Work out the finished part from the listing and answer in its coordinate system (mm). A direction names the side the tool comes from. Round coordinates to 2 decimals unless told otherwise and drop trailing zeros. Write each loop counter-clockwise with the first axis right and the second up, starting at its lowest first coordinate (ties: lowest second). Pieces come first, ordered by that corner, then holes.
from build123d import *

# Parameters (mm, degrees)
ESQUISSE1_R             = 1.6
BOSS_EXTRU_1_DEPTH      = 10.1
ESQUISSE2_R             = 32.8
BOSS_EXTRU_2_DEPTH      = 21
ENL_V_MAT_EXTRU_1_DEPTH = 3.5
ESQUISSE4_R             = 32.8
BOSS_EXTRU_3_DEPTH      = 3.5
ESQUISSE5_R             = 16
BOSS_EXTRU_4_DEPTH      = 20.7
ESQUISSE8_R             = 5
BOSS_EXTRU_7_DEPTH      = 5.5
SKETCH6_R               = 34.35
BOSS_EXTRUDE3_DEPTH     = 9.3
CUT_EXTRUDE1_REACH      = 83.139
CUT_EXTRUDE1_END_RADIUS = 32.8
SKETCH5_R               = 5.25
ESQUISSE6_R             = 1
BOSS_EXTRU_5_DEPTH      = 7.7
BOSS_EXTRUDE4_DEPTH     = 10.6


with BuildPart() as part:
    # Esquisse1 → Boss.-Extru.1 (new body)
    with BuildSketch(Plane.XY):
        with BuildLine():
            ThreePointArc((-56.3, -16.861494596), (-60.528670487, -14.599558136), (-64.01, -11.301322931))
            ThreePointArc((-64.01, -11.301322931), (-65, 0), (-64.01, 11.301322931))
            ThreePointArc((-64.01, 11.301322931), (-60.528670487, 14.599558136), (-56.3, 16.861494596))
            Line((-56.3, 16.861494596), (-39.156313776, 23.266930519))
            ThreePointArc((-39.156313776, 23.266930519), (-36.515940127, 29.057304168), (-30.725566478, 26.416930519))
            Line((-30.725566478, 26.416930519), (-12.425, 33.254614341))
            ThreePointArc((-12.425, 33.254614341), (1.381675102, 35.473102119), (14.973963383, 32.187426436))
            Line((14.973963383, 32.187426436), (20.756023105, 34.801647207))
            ThreePointArc((20.756023105, 34.801647207), (24.347774736, 34.238511045), (26, 31))
            Line((26, 31), (25.359978077, 24.841930519))
            ThreePointArc((25.359978077, 24.841930519), (35.5, 0), (25.359978077, -24.841930519))
            Line((25.359978077, -24.841930519), (26, -31))
            ThreePointArc((26, -31), (24.347774736, -34.238511045), (20.756023105, -34.801647207))
            Line((20.756023105, -34.801647207), (14.973963383, -32.187426436))
            ThreePointArc((14.973963383, -32.187426436), (1.381675102, -35.473102119), (-12.425, -33.254614341))
            Line((-12.425, -33.254614341), (-30.725566478, -26.416930519))
            ThreePointArc((-30.725566478, -26.416930519), (-36.515940127, -29.057304168), (-39.156313776, -23.266930519))
            Line((-39.156313776, -23.266930519), (-56.3, -16.861494596))
        make_face()
        with Locations((-35, -25)):
            Circle(ESQUISSE1_R, mode=Mode.SUBTRACT)
        with Locations((22, 31)):
            Circle(ESQUISSE1_R, mode=Mode.SUBTRACT)
        with Locations((-35, 25)):
            Circle(ESQUISSE1_R, mode=Mode.SUBTRACT)
        with Locations((22, -31)):
            Circle(ESQUISSE1_R, mode=Mode.SUBTRACT)
    extrude(amount=BOSS_EXTRU_1_DEPTH)

    # Esquisse2 → Boss.-Extru.2 (add)
    with BuildSketch(Plane.XY.offset(10.1)):
        with Locations(Location((0, 0, 0), (0, 0, 180))):
            Circle(ESQUISSE2_R)
    extrude(amount=BOSS_EXTRU_2_DEPTH)

    # Esquisse3 → Enl_v. mat.-Extru.1 (cut)
    with BuildSketch(Plane.XY.offset(10.1)):
        with BuildLine():
            Line((-55.775, -15.456370046), (-36.849687238, -22.527479296))
            ThreePointArc((-36.849687238, -22.527479296), (-35.990940127, -27.652179619), (-31.982193016, -24.346132644))
            Line((-31.982193016, -24.346132644), (-11.9, -31.849489792))
            ThreePointArc((-11.9, -31.849489792), (1.664031028, -33.959255009), (14.956816294, -30.533484019))
            Line((14.956816294, -30.533484019), (21.291141631, -33.397398551))
            ThreePointArc((21.291141631, -33.397398551), (23.468656713, -33.023128137), (24.499056843, -31.06866508))
            Line((24.499056843, -31.06866508), (23.79417774, -24.286562245))
            ThreePointArc((23.79417774, -24.286562245), (34, 0), (23.79417774, 24.286562245))
            Line((23.79417774, 24.286562245), (24.499056843, 31.06866508))
            ThreePointArc((24.499056843, 31.06866508), (23.468656713, 33.023128137), (21.291141631, 33.397398551))
            Line((21.291141631, 33.397398551), (14.956816294, 30.533484019))
            ThreePointArc((14.956816294, 30.533484019), (1.664031028, 33.959255009), (-11.9, 31.849489792))
            Line((-11.9, 31.849489792), (-31.982193016, 24.346132644))
            ThreePointArc((-31.982193016, 24.346132644), (-35.990940127, 27.652179619), (-36.849687238, 22.527479296))
            Line((-36.849687238, 22.527479296), (-55.775, 15.456370046))
            ThreePointArc((-55.775, 15.456370046), (-59.496201473, 13.493411636), (-62.6, 10.653168543))
            ThreePointArc((-62.6, 10.653168543), (-63.5, 0), (-62.6, -10.653168543))
            ThreePointArc((-62.6, -10.653168543), (-59.496201473, -13.493411636), (-55.775, -15.456370046))
        make_face()
    extrude(amount=-ENL_V_MAT_EXTRU_1_DEPTH, mode=Mode.SUBTRACT)


with BuildPart() as enl_v_mat_extru_1_piece_1:
    # of the separate pieces the step leaves, piece 1, a body of its own (enl_v_mat_extru_1_pieces)
    add(part.part.solids().sort_by_distance((-32.8, 0, 10.1))[0])



with BuildPart() as enl_v_mat_extru_1_piece_2:
    # of the separate pieces the step leaves, piece 2, a body of its own (enl_v_mat_extru_1_pieces)
    add(part.part.solids().sort_by_distance((-64.01, 11.301322931, 0))[0])


with BuildPart() as enl_v_mat_extru_1_piece_1_1:
    add(enl_v_mat_extru_1_piece_1.part)

    add(enl_v_mat_extru_1_piece_2.part)  # Boss.-Extru.3 merges Enl_v. mat.-Extru.1 piece 2
    # Esquisse4 → Boss.-Extru.3 (add)
    with BuildSketch(Plane(origin=(0, 0, 10.1), x_dir=(-1, 0, 0), z_dir=(0, 0, -1))):
        with Locations(Location((0, 0, 0), (0, 0, 180))):
            Circle(ESQUISSE4_R)
    extrude(amount=BOSS_EXTRU_3_DEPTH)

    # Esquisse5 → Boss.-Extru.4 (add)
    with BuildSketch(Plane(origin=(0, 0, 0), x_dir=(-1, 0, 0), z_dir=(0, 0, -1))):
        with Locations(Location((50, 0, 0), (0, 0, 336.653490915))):
            Circle(ESQUISSE5_R)
    extrude(amount=BOSS_EXTRU_4_DEPTH)

    # Esquisse8 → Boss.-Extru.7 (add)
    with BuildSketch(Plane.XY.offset(6.6)):
        with Locations((-50, 0)):
            Circle(ESQUISSE8_R)
    extrude(amount=BOSS_EXTRU_7_DEPTH)

    # Sketch6 → Boss-Extrude3 (add)
    with BuildSketch(Plane.XY.offset(6.6)):
        with Locations(Location((0, 0, 0), (0, 0, 118.673428071))):
            Circle(SKETCH6_R)
    extrude(amount=BOSS_EXTRUDE3_DEPTH)

    # Cut-Extrude1: up to this cylinder (the profile starts inside it)
    cut_extrude1_end = Plane(origin=(0, 0, 21.7), z_dir=(0, 0, 1)) * Cylinder(CUT_EXTRUDE1_END_RADIUS, 232.878, mode=Mode.PRIVATE)
    # Sketch5 → Cut-Extrude1 (cut, up to the surface)
    with BuildSketch(Plane(origin=(0, 0, 0), x_dir=(1, 0, 0), z_dir=(0, 1, 0)), mode=Mode.PRIVATE) as cut_extrude1_sk1:
        with Locations(Location((-18, -21.7, 0), (0, 0, 270))):
            Circle(SKETCH5_R)
    cut_extrude1_tool1 = extrude(cut_extrude1_sk1.sketch, amount=-CUT_EXTRUDE1_REACH, mode=Mode.PRIVATE) & cut_extrude1_end
    add(cut_extrude1_tool1.solids().sort_by_distance((-18, 0, 21.7))[0], mode=Mode.SUBTRACT)
    # Sketch5 → Cut-Extrude1 (cut, up to the surface)
    with BuildSketch(Plane(origin=(0, 0, 0), x_dir=(1, 0, 0), z_dir=(0, 1, 0)), mode=Mode.PRIVATE) as cut_extrude1_sk2:
        with BuildLine():
            Line((14.75, -16.45), (21.25, -16.45))
            ThreePointArc((21.25, -16.45), (26.5, -21.7), (21.25, -26.95))
            Line((21.25, -26.95), (14.75, -26.95))
            ThreePointArc((14.75, -26.95), (9.5, -21.7), (14.75, -16.45))
        make_face()
    cut_extrude1_tool2 = extrude(cut_extrude1_sk2.sketch, amount=-CUT_EXTRUDE1_REACH, mode=Mode.PRIVATE) & cut_extrude1_end
    add(cut_extrude1_tool2.solids().sort_by_distance((18, 0, 21.7))[0], mode=Mode.SUBTRACT)

    # Esquisse6 → Boss.-Extru.5 (add)
    # profile 1 of 4: a face of its own
    with BuildSketch(Plane(origin=(0, 0, 0), x_dir=(-1, 0, 0), z_dir=(0, 0, -1))):
        Polygon((-20.489225606, -29.008126327), (-22.969626005, -28.695694159), (-24.480400399, -30.687567832), (-23.510774394, -32.991873673), (-21.030373995, -33.304305841), (-19.519599601, -31.312432168), align=None)
        with Locations((-22, -31)):
            Circle(ESQUISSE6_R, mode=Mode.SUBTRACT)
    # profile 2 of 4: a face of its own
    with BuildSketch(Plane(origin=(0, 0, 0), x_dir=(-1, 0, 0), z_dir=(0, 0, -1))):
        Polygon((36.086835018, -22.748602735), (33.593650283, -22.933074633), (32.506815266, -25.184471898), (33.913164982, -27.251397265), (36.406349717, -27.066925367), (37.493184734, -24.815528102), align=None)
        with Locations((35, -25)):
            Circle(ESQUISSE6_R, mode=Mode.SUBTRACT)
    # profile 3 of 4: a face of its own
    with BuildSketch(Plane(origin=(0, 0, 0), x_dir=(-1, 0, 0), z_dir=(0, 0, -1))):
        Polygon((36.720274889, 26.814016072), (34.289153443, 27.396809791), (32.568878555, 25.582793719), (33.279725111, 23.185983928), (35.710846557, 22.603190209), (37.431121445, 24.417206281), align=None)
        with Locations((35, 25)):
            Circle(ESQUISSE6_R, mode=Mode.SUBTRACT)
    # profile 4 of 4: a face of its own
    with BuildSketch(Plane(origin=(0, 0, 0), x_dir=(-1, 0, 0), z_dir=(0, 0, -1))):
        Polygon((-19.952160425, 32.43399898), (-22.217959758, 33.490480585), (-24.265799333, 32.056481605), (-24.047839575, 29.56600102), (-21.782040242, 28.509519415), (-19.734200667, 29.943518395), align=None)
        with Locations((-22, 31)):
            Circle(ESQUISSE6_R, mode=Mode.SUBTRACT)
    extrude(amount=BOSS_EXTRU_5_DEPTH)

    # Sketch7 → Boss-Extrude4 (add)
    with BuildSketch(Plane(origin=(0, 0, -20.7), x_dir=(-1, 0, 0), z_dir=(0, 0, -1))):
        with BuildLine():
            Line((45.459437733, 15.342206305), (41.857967445, 21.344656785))
            Line((41.857967445, 21.344656785), (38.427995742, 19.286673763))
            Line((38.427995742, 19.286673763), (34.998024039, 17.228690741))
            Line((34.998024039, 17.228690741), (38.599494327, 11.226240261))
            ThreePointArc((38.599494327, 11.226240261), (41.768067913, 13.719886811), (45.459437733, 15.342206305))
        make_face()
    extrude(amount=-BOSS_EXTRUDE4_DEPTH)


solid = enl_v_mat_extru_1_piece_1_1.part
Q1. Find the intervals of material crossed by L1, parallel to Y at x = -18.5, z = 9.5; L2, parallel to X at y = 25, z = 3; L3, parallel to X at y = -6, z = 23, in increasing order.
Q2. Find section B-B (y = -9). Determine the outline of the cut face in (x, z), plus the area to 3 significant figures.
Q3. The mould has two halves that part along Y. Classify faces 1 (the face through (26.5, -9.5, 21.6)), 2 (the face through (-59.448, 13.527, 8.374)), 3 (the face through (-63.5, 0.1, 8.4)), 4 (the face through (-65, 0, 5)): +Y half, -Y half, draft (parallel to the pull), parting line (faces both ways), or undercut.
Q4. Given pin 1 (8.5 mm diameter, centred on x = -20.5, z = 24, fed in from -Y); pin 2 (1 mm diameter, centred on y = 10, z = 20.5, fed in from +X); pin 3 (8 mm diameter, centred on y = 13, z = -13, fed in from -X); pin 4 (1.6 mm diameter, centred on x = -35, y = -25, fed in from +Z), each flat-ended and moving along its own axis, determine where each tip first touches the part or whether it passes through.
Q5. A tool of negligible diameter and unlimited length cuts with its end or side. For faces 5 (the face through (23.526, -30.519, 3.254)), 6 (the face through (23.23, 32.78, -3.8)), 7 (the face through (-18, 0, 22)), 8 (the face through (-37.08, 25.6, -3.8)), 9 (the face through (-21.7, 29.79, 4.98)), from which of +Z, -Z, +X, -X, +Y, -Y can it reach the whole face along a straight path? Write none if from no direction.
Q6. Find section C-C (x = 0). Determine the outline of the cut face in (y, z).
Q7. Find section A-A (z = 2.5). Determine the outline of the cut face in (x, y) (1 decimal), plus the area to 3 significant figures.
Q8. Find section D-D (x = 29). Determine the outline of the cut face in (y, z), plus the area to 3 significant figures.
Report:
1. L1: y = -30.98 to -29.38, -28.94 to 28.94, 29.38 to 30.98
1. L2: x = -39.44 to -36.6, -33.4 to 25.38
1. L3: x = -32.25 to -23.09, -12.91 to 9.66, 26.34 to 32.25
2. outline: (-64.37, 0) - (-63.23, 0) - (-63.23, -20.7) - (-36.77, -20.7) - (-36.77, 0) - (34.34, 0) - (34.34, 10.1) - (33.15, 10.1) - (33.15, 15.9) - (31.54, 15.9) - (31.54, 31.1) - (-31.54, 31.1) - (-31.54, 15.9) - (-33.15, 15.9) - (-33.15, 6.6) - (-62.86, 6.6) - (-62.86, 10.1) - (-64.37, 10.1) - close; hole circle Ø10.5 at (-18, 21.7); hole (14.75, 16.45) - (21.25, 16.45) arc R5.25 ccw to (21.25, 26.95) - (14.75, 26.95) arc R5.25 ccw to start
2. area: 2,540 mm2
3. face 1: draft
3. face 2: undercut
3. face 3: undercut
3. face 4: parting line
4. pin 1: stops at y = -27.8
4. pin 2: stops at x = 31.39
4. pin 3: stops at x = -63.23
4. pin 4: passes through
5. face 5: +Z
5. face 6: -Z, +X, +Y
5. face 7: -Y
5. face 8: -Z, -X, +Y
5. face 9: +Z, -Z, +Y
6. outline: (-35.5, 0) - (35.5, 0) - (35.5, 10.1) - (34.35, 10.1) - (34.35, 15.9) - (32.8, 15.9) - (32.8, 31.1) - (-32.8, 31.1) - (-32.8, 15.9) - (-34.35, 15.9) - (-34.35, 10.1) - (-35.5, 10.1) - close
7. outline: (-64, -11.3) arc R18 ccw to (-56.3, -16.9) - (-39.2, -23.3) arc R4.5 ccw to (-30.7, -26.4) - (-12.4, -33.3) arc R35.5 ccw to (15, -32.2) - (20.8, -34.8) arc R4 ccw to (26, -31) - (25.4, -24.8) arc R35.5 ccw to (25.4, 24.8) - (26, 31) arc R4 ccw to (20.8, 34.8) - (15, 32.2) arc R35.5 ccw to (-12.4, 33.3) - (-30.7, 26.4) arc R4.5 ccw to (-39.2, 23.3) - (-56.3, 16.9) arc R18 ccw to (-64, 11.3) arc R65 ccw to start; hole circle Ø3.2 at (-35, -25); hole circle Ø3.2 at (-35, 25); hole circle Ø3.2 at (22, -31); hole circle Ø3.2 at (22, 31)
7. area: 5,420 mm2
8. outline: (-20.48, 0) - (20.48, 0) - (20.48, 10.1) - (18.41, 10.1) - (18.41, 15.9) - (15.32, 15.9) - (15.32, 31.1) - (-15.32, 31.1) - (-15.32, 15.9) - (-18.41, 15.9) - (-18.41, 10.1) - (-20.48, 10.1) - close
8. area: 1,090 mm2
